The model under review builds one solid part; all positions refer to its coordinate system, in mm. Round coordinates to 2 decimals unless told otherwise and drop trailing zeros. Write each loop counter-clockwise with the first axis right and the second up, starting at its lowest first coordinate (ties: lowest second). Pieces come first, ordered by that corner, then holes. Notation, with made-up numbers: (56.5, 51.25) - (81.5, 51.25) arc R18 ccw to (81.5, 74.25) - close; hole circle Ø9 at (48, 9.25). An arc over 180 degrees is marked (long way). Return JSON: item names as keys, results as strings.
from build123d import *

# Parameters (mm, degrees)
BOSS_EXTRU_1_DEPTH      = 3
ESQUISSE2_R             = 1.25
ENL_V_MAT_EXTRU_1_DEPTH = 10


with BuildPart() as part:
    # Esquisse1 → Boss.-Extru.1 (new body)
    with BuildSketch(Plane.XY):
        Polygon((-56.390469464, -21.033092325), (-56.390469464, -51.033092325), (163.609530536, -51.033092325), (163.609530536, -21.033092325), (153.609530536, -21.033092325), (153.609530536, -11.033092325), (156.009530536, -11.033092325), (156.009530536, 138.966907675), (153.609530536, 138.966907675), (153.609530536, 141.366907675), (-46.390469464, 141.366907675), (-46.390469464, 138.966907675), (-48.790469464, 138.966907675), (-48.790469464, -11.033092325), (-46.390469464, -11.033092325), (-46.390469464, -21.033092325), align=None)
    extrude(amount=BOSS_EXTRU_1_DEPTH)

    # Esquisse2 → Enlèv. mat.-Extru.1 (cut)
    with BuildSketch(Plane.XY.offset(3)):
        with Locations((160.319530536, -34.033092325)):
            Circle(ESQUISSE2_R)
        with Locations((112.059530536, -34.033092325)):
            Circle(ESQUISSE2_R)
        with Locations((160.319530536, -44.193092325)):
            Circle(ESQUISSE2_R)
        with Locations((112.059530536, -44.193092325)):
            Circle(ESQUISSE2_R)
        with Locations((-4.840469464, -44.193092325)):
            Circle(ESQUISSE2_R)
        with Locations((-53.100469464, -44.193092325)):
            Circle(ESQUISSE2_R)
        with Locations((-4.840469464, -34.033092325)):
            Circle(ESQUISSE2_R)
        with Locations((-53.100469464, -34.033092325)):
            Circle(ESQUISSE2_R)
    extrude(amount=-ENL_V_MAT_EXTRU_1_DEPTH, mode=Mode.SUBTRACT)


solid = part.part
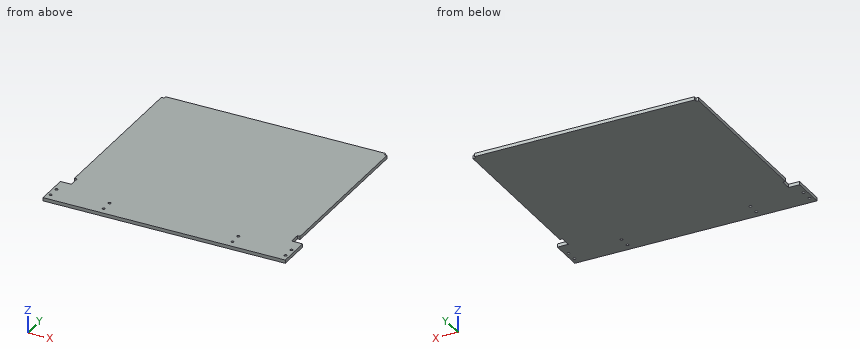
(1) Clearance check with flat-ended pins moving along their axes: pin 1 Ø3 at (x, y) = (112.06, -34.03) entering from +Z; pin 2 Ø0.7 at (x, z) = (154.5, 1.5) entering from +Y; pin 3 Ø1.5 at (x, z) = (-53, 1.5) entering from +Y; pin 4 Ø1.2 at (y, z) = (140, 1.5) entering from +X. State where each tip first meets the part, or that it passes through.
Filled in:
{"pin 1": "stops at z = 3", "pin 2": "stops at y = 138.97", "pin 3": "stops at y = -21.03", "pin 4": "stops at x = 153.61"}
(2) Add section B-B (y = -15). Write out the cut boundary in (x, z).
Filled in:
{"outline": "(-46.39, 0) - (153.61, 0) - (153.61, 3) - (-46.39, 3) - close"}
(3) Add section C-C (y = 45.5). Write out the cut boundary in (x, z), plus the area to 3 significant figures.
Filled in:
{"outline": "(-48.79, 0) - (156.01, 0) - (156.01, 3) - (-48.79, 3) - close", "area": "614 mm2"}
(4) Wall thickness on line 1 (X direction, y = -9, z = 1.95); line 2 (X direction, y = -19, z = 1.8): over which ranges is each line inside the solid? List them lowest first.
Filled in:
{"line 1": "x = -48.79 to 156.01", "line 2": "x = -46.39 to 153.61"}
(5) Add section A-A (z = 0.7). Give the number of separate pieces and of enclosed holes in the cut face, plus the area to 3 significant figures.
Filled in:
{"separate pieces": "1", "enclosed holes": "8", "area": "39,800 mm2"}
